from build123d import *

# Parameters (mm, degrees)
SKETCH_1_R          = 13
EXTRUDE_634_DEPTH   = 7.5
SKETCH_2_W          = 2408.049034164
SKETCH_2_H          = 7.5
EXTRUDE_1_DEPTH     = 89
SKETCH_3_W          = 80
SKETCH_3_H          = 240
EXTRUDE_2_DEPTH     = 16
SKETCH_4_R          = 13
CUT_EXTRUDE_1_DEPTH = 1308.983562588


with BuildPart() as part:
    # 草图1 → Extrude 634 (new body)
    with BuildSketch(Plane.XY):
        Polygon((-1205, 0), (1205, 0), (1270, 50), (1270, 250), (1205, 300), (-1205, 300), (-1270, 250), (-1270, 50), align=None)
        with Locations((-1220, 230)):
            Circle(SKETCH_1_R, mode=Mode.SUBTRACT)
        with Locations((-1220, 150)):
            Circle(SKETCH_1_R, mode=Mode.SUBTRACT)
        with Locations((-1140, 230)):
            Circle(SKETCH_1_R, mode=Mode.SUBTRACT)
        with Locations((-1140, 150)):
            Circle(SKETCH_1_R, mode=Mode.SUBTRACT)
        with Locations((-1060, 230)):
            Circle(SKETCH_1_R, mode=Mode.SUBTRACT)
        with Locations((-1060, 150)):
            Circle(SKETCH_1_R, mode=Mode.SUBTRACT)
        with Locations((-980, 150)):
            Circle(SKETCH_1_R, mode=Mode.SUBTRACT)
        with Locations(Location((-1060, 70, 0), (0, 0, 180))):
            Circle(SKETCH_1_R, mode=Mode.SUBTRACT)
        with Locations(Location((-1140, 70, 0), (0, 0, 180))):
            Circle(SKETCH_1_R, mode=Mode.SUBTRACT)
        with Locations(Location((-1220, 70, 0), (0, 0, 180))):
            Circle(SKETCH_1_R, mode=Mode.SUBTRACT)
        with Locations((1220, 70)):
            Circle(SKETCH_1_R, mode=Mode.SUBTRACT)
        with Locations((1140, 70)):
            Circle(SKETCH_1_R, mode=Mode.SUBTRACT)
        with Locations((1060, 70)):
            Circle(SKETCH_1_R, mode=Mode.SUBTRACT)
        with Locations(Location((980, 150, 0), (0, 0, 180))):
            Circle(SKETCH_1_R, mode=Mode.SUBTRACT)
        with Locations(Location((1060, 150, 0), (0, 0, 180))):
            Circle(SKETCH_1_R, mode=Mode.SUBTRACT)
        with Locations(Location((1060, 230, 0), (0, 0, 180))):
            Circle(SKETCH_1_R, mode=Mode.SUBTRACT)
        with Locations(Location((1140, 150, 0), (0, 0, 180))):
            Circle(SKETCH_1_R, mode=Mode.SUBTRACT)
        with Locations(Location((1140, 230, 0), (0, 0, 180))):
            Circle(SKETCH_1_R, mode=Mode.SUBTRACT)
        with Locations(Location((1220, 150, 0), (0, 0, 180))):
            Circle(SKETCH_1_R, mode=Mode.SUBTRACT)
        with Locations(Location((1220, 230, 0), (0, 0, 180))):
            Circle(SKETCH_1_R, mode=Mode.SUBTRACT)
    extrude(amount=-EXTRUDE_634_DEPTH)

    # 草图2 → 凸台-拉伸1 (add)
    with BuildSketch(Plane.XY):
        with Locations((-0.975482918, 296.25)):
            Rectangle(SKETCH_2_W, SKETCH_2_H)
        with Locations((-0.975482918, 3.75)):
            Rectangle(SKETCH_2_W, SKETCH_2_H)
    extrude(amount=EXTRUDE_1_DEPTH)

    # 草图3 → 凸台-拉伸2 (add)
    with BuildSketch(Plane(origin=(0, 0, -7.5), x_dir=(-1, 0, 0), z_dir=(0, 0, -1))):
        with Locations((-580, 150)):
            Rectangle(SKETCH_3_W, SKETCH_3_H)
        with Locations((-180, 150)):
            Rectangle(SKETCH_3_W, SKETCH_3_H)
        with Locations((180, 150)):
            Rectangle(SKETCH_3_W, SKETCH_3_H)
        with Locations((580, 150)):
            Rectangle(SKETCH_3_W, SKETCH_3_H)
    extrude(amount=EXTRUDE_2_DEPTH)

    # 草图4 → 切除-拉伸1 (cut, through all)
    with BuildSketch(Plane.XY):
        with Locations((-580, 230)):
            Circle(SKETCH_4_R)
        with Locations((-580, 150)):
            Circle(SKETCH_4_R)
        with Locations((-180, 230)):
            Circle(SKETCH_4_R)
        with Locations((-180, 150)):
            Circle(SKETCH_4_R)
        with Locations(Location((-180, 70, 0), (0, 0, 180))):
            Circle(SKETCH_4_R)
        with Locations(Location((-580, 70, 0), (0, 0, 180))):
            Circle(SKETCH_4_R)
        with Locations((580, 70)):
            Circle(SKETCH_4_R)
        with Locations((180, 70)):
            Circle(SKETCH_4_R)
        with Locations(Location((180, 150, 0), (0, 0, 180))):
            Circle(SKETCH_4_R)
        with Locations(Location((180, 230, 0), (0, 0, 180))):
            Circle(SKETCH_4_R)
        with Locations(Location((580, 150, 0), (0, 0, 180))):
            Circle(SKETCH_4_R)
        with Locations(Location((580, 230, 0), (0, 0, 180))):
            Circle(SKETCH_4_R)
    extrude(amount=-CUT_EXTRUDE_1_DEPTH, mode=Mode.SUBTRACT)


solid = part.part
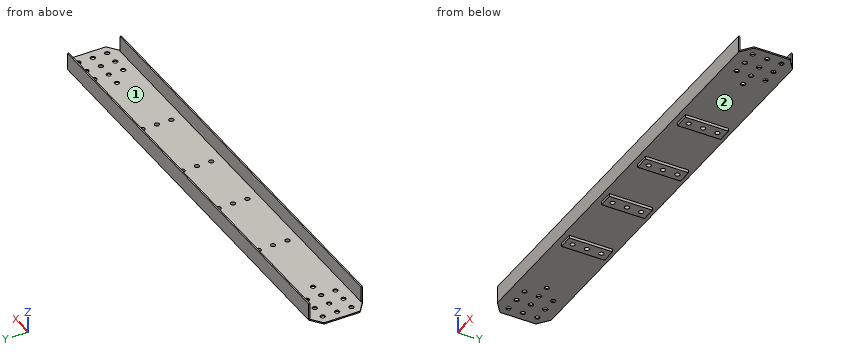
The model under review builds one solid part; all positions refer to its coordinate system, in mm. Face numbers are marked on the shaded views. Coordinates: 2 decimals unless noted, no trailing zeros. Loops run counter-clockwise (first coordinate to the right, second up) from the corner with the lowest first, then second, coordinate; pieces in that order, holes last. Notation, with made-up numbers: M 44.25,-5.5 L 85.25,-5.5 A17 ccw 85.25,16.5 Z; hole C 79,84 d1. An arc over 180 degrees is marked long. Put each result on its own line as item: value. Start each with the question number.
Q1. The part is to be moulded in two halves that separate along X. For the marked faces 1 and 2, say which applies: +X half, -X half, draft (parallel to the pull), parting line (faces both ways), or undercut.
Q2. Clearance check with flat-ended pins moving along their axes: pin 1 (23.5 mm diameter, centred on x = 580, y = 230, fed in from +Z); pin 2 (6 mm diameter, centred on y = 295.5, z = 60, fed in from -X); pin 3 (3 mm diameter, centred on x = -100.5, y = 72.5, fed in from +Z); pin 4 (12 mm diameter, centred on x = -716.5, y = 246.5, fed in from -Z). State where each tip first meets the part, or that it passes through.
Q3. Wall thickness on line 1 (X direction, y = 190.5, z = -12); line 2 (Y direction, x = -1038, z = 62); line 3 (Y direction, x = 580, z = -16.5): over which ranges is each line inside the solid? List them lowest first.
Q4. Add section A-A (z = 59). Write out the cut boundary in (x, y), and give its area (3 significant figures).
Q5. Add section B-B (x = -685). Write out the cut boundary in (y, z), and give its area (4 significant figures).
Answers:
1. face 1: draft
1. face 2: undercut
2. pin 1: passes through
2. pin 2: stops at x = -1205
2. pin 3: stops at z = 0
2. pin 4: stops at z = -7.5
3. line 1: x = -620 to -540, -220 to -140, 140 to 220, 540 to 620
3. line 2: y = 0 to 7.5, 292.5 to 300
3. line 3: y = 30 to 57, 83 to 137, 163 to 217, 243 to 270
4. outline: M -1205,0 L 1203.05,0 L 1203.05,7.5 L -1205,7.5 Z; M -1205,292.5 L 1203.05,292.5 L 1203.05,300 L -1205,300 Z
4. area: 36,100 mm^2
5. outline: M 0,-7.5 L 300,-7.5 L 300,89 L 292.5,89 L 292.5,0 L 7.5,0 L 7.5,89 L 0,89 Z
5. area: 3,585 mm^2
